Autodesk Fusion 360 part; units mm, degrees
sketch "Sketch1" plane through (0, 0, 0) normal (0, 0, 1) x (1, 0, 0)
  circle A0 centre (50, 25) radius 15
  dimension "d1" = 30
extrude "Extrude1" add sketch "Sketch1" along normal blind 60
sketch "Sketch2" plane through (0, 0, 60) normal (0, 0, 1) x (-1, 0, 0)
  circle A0 centre (-50, -25) radius 15
  circle A1 centre (-50, -25) radius 2.5
  dimension "d4" = 5
extrude "Extrude2" cut sketch "Sketch2" against normal blind 55 contours A1
sketch "Sketch3" plane through (0, 0, 60) normal (0, 0, 1) x (-1, 0, 0)
  circle A0 centre (-50, -25) radius 2.5
  circle A1 centre (-50, -25) radius 15
  circle A2 centre (-50, -25) radius 12
  dimension "d7" = 24
extrude "Extrude3" cut sketch "Sketch3" against normal blind 55 contours A1
sketch "Sketch4" plane through (0, 0, 60) normal (0, 0, 1) x (-1, 0, 0)
  circle A0 centre (-50, -25) radius 12
  circle A1 centre (-50, -25) radius 2.5
  circle A2 centre (-50, -25) radius 15
  dimension "d10" = 30
extrude "Extrude4" add sketch "Sketch4" against normal blind 5 contours A2
extrude "Extrude5" cut 1 faces at (63.9442, 25.7452, 5) along direction (0, 0, 1) blind 55
extrude "Extrude6" add 1 faces at (41.2207, 25.7204, 60) along direction (0, 0, -1) blind 55
extrude "Extrude7" add 1 faces at (41.2207, 25.7204, 60) along direction (0, 0, 1) blind 35
sketch "Sketch5" plane through (0, 0, 95) normal (0, 0, 1) x (-1, 0, 0)
  circle A0 centre (-50, -25) radius 12
  circle A1 centre (-50, -25) radius 2.5
  circle A2 centre (-50, -25) radius 2.65
  dimension "d19" = 5.3
extrude "Extrude8" cut sketch "Sketch5" against normal blind 90 contours A2
sketch "Sketch6" plane through (0, 0, 95) normal (0, 0, 1) x (-1, 0, 0)
  circle A0 centre (-50, -25) radius 2.65
  circle A1 centre (-50, -25) radius 12
  circle A2 centre (-50, -25) radius 15
  dimension "d22" = 30
extrude "Extrude9" add sketch "Sketch6" along normal blind 5 contours A1 | A2
Work out the finished part from the listing and answer in its coordinate system (mm). A direction names the side the tool comes from. Give positions to 0.01 mm unless a question says otherwise; leave off trailing zeros. Write each loop counter-clockwise with the first axis right and the second up, starting at its lowest first coordinate (ties: lowest second). Pieces come first, ordered by that corner, then holes. Notation, with made-up numbers: (-10, 56.25) -> (15, 56.25) arc R24 cw to (15, 92.25) -> close; hole circle Ø8 at (-14.75, 74). An arc over 180 degrees is marked (long way). Write each question's results on one line, items separated by ' | '.
1. Straight lines are drawn through the part: L1, parallel to Y at x = 50, z = 70.5; L2, parallel to X at y = 25, z = 34; L3, parallel to Z at x = 60.75, y = 19.25. For each, find the intervals that lie inside material, in ascending order.
Data:
L1: 13 to 22.35, 27.65 to 37 | L2: 38 to 47.35, 52.65 to 62 | L3: 0 to 5, 95 to 100
2. Each of these flat-tipped pins is pushed along its axis until it touches: pin 1 Ø6 at (x, z) = (59.5, 55) entering from -Y; pin 2 Ø12 at (x, z) = (39, 33) entering from +Y; pin 3 Ø6 at (y, z) = (21, 51) entering from -X. Where does it stop, or does it pass through?
Data:
pin 1: y = 14.91 | pin 2: y = 35.91 | pin 3: x = 38.04
3. Find section C-C on x = 50. Determine the outline of the cut face in (y, z), and give its area (3 significant figures).
Data:
outline: (10, 0) -> (40, 0) -> (40, 5) -> (37, 5) -> (37, 95) -> (40, 95) -> (40, 100) -> (27.65, 100) -> (27.65, 5) -> (22.35, 5) -> (22.35, 100) -> (10, 100) -> (10, 95) -> (13, 95) -> (13, 5) -> (10, 5) -> close | area: 1,960 mm^2
4. Determine the mould class of faces 4 (the cylindrical face through (62, 16, 97)), 5 (the flat face through (50, 25, 0)), 6 (the flat face through (57, 15, 95)), 7 (the flat face through (47, 25, 100)) for opening direction Z: +Z half, -Z half, draft (parallel to the pull), parting line (faces both ways), or undercut.
Data:
face 4: draft | face 5: -Z half | face 6: undercut | face 7: +Z half
5. A tool of negligible diameter and unlimited length cuts with its end or side. For faces 1 (the flat face through (50, 25, 5)), 2 (the cylindrical face through (59.523, 17.698, 49.37)), 3 (the cylindrical face through (38, 34, 2)), from which of +Z, -Z, +X, -X, +Y, -Y can it reach the whole face along a straight path? Write none if from no direction.
Data:
face 1: +Z | face 2: none | face 3: +Z, -Z
6. Find section B-B on y = 25. Determine the outline of the cut face in (x, z).
Data:
outline: (35, 0) -> (65, 0) -> (65, 5) -> (62, 5) -> (62, 95) -> (65, 95) -> (65, 100) -> (52.65, 100) -> (52.65, 5) -> (47.35, 5) -> (47.35, 100) -> (35, 100) -> (35, 95) -> (38, 95) -> (38, 5) -> (35, 5) -> close
7. Find section D-D on x = 40. Determine the outline of the cut face in (y, z), and give its area (3 significant figures).
Data:
outline: (13.82, 0) -> (36.18, 0) -> (36.18, 5) -> (31.63, 5) -> (31.63, 95) -> (36.18, 95) -> (36.18, 100) -> (13.82, 100) -> (13.82, 95) -> (18.37, 95) -> (18.37, 5) -> (13.82, 5) -> close | area: 1,420 mm^2
8. Find section A-A on z = 14.5. Determine the outline of the cut face in (x, y).
Data:
outline: circle Ø24 at (50, 25); hole circle Ø5.3 at (50, 25)
